from build123d import *

# Parameters (mm, degrees)
ESQUISSE2_R             = 35
ESQUISSE2_R_2           = 5
ESQUISSE2_R_3           = 3.16227766
BASE_EXTRUSION_DEPTH    = 8
ESQUISSE3_R             = 17.492855685
ESQUISSE3_R_2           = 15
BOSS_EXTRU_1_DEPTH      = 20
ESQUISSE4_W             = 72
ESQUISSE4_H             = 33
ENL_V_MAT_EXTRU_2_DEPTH = 57.868268832


with BuildPart() as part:
    # Esquisse2 → Base-Extrusion (new body)
    with BuildSketch(Plane(origin=(0, 0, 0), x_dir=(1, 0, 0), z_dir=(0, 1, 0))):
        Circle(ESQUISSE2_R)
        Circle(ESQUISSE2_R_2, mode=Mode.SUBTRACT)
        with Locations((-28, 0)):
            Circle(ESQUISSE2_R_3, mode=Mode.SUBTRACT)
        with Locations(Location((0, 28, 0), (0, 0, 270))):
            Circle(ESQUISSE2_R_3, mode=Mode.SUBTRACT)
        with Locations((0, -28)):
            Circle(ESQUISSE2_R_3, mode=Mode.SUBTRACT)
        with Locations((28, 0)):
            Circle(ESQUISSE2_R_3, mode=Mode.SUBTRACT)
    extrude(amount=BASE_EXTRUSION_DEPTH)

    # Esquisse3 → Boss.-Extru.1 (add)
    with BuildSketch(Plane(origin=(0, 8, 0), x_dir=(-1, 0, 0), z_dir=(0, 1, 0))):
        Circle(ESQUISSE3_R)
        Circle(ESQUISSE3_R_2, mode=Mode.SUBTRACT)
    extrude(amount=BOSS_EXTRU_1_DEPTH)

    # Esquisse4 → Enlèv. mat.-Extru.2 (cut, through all)
    with BuildSketch(Plane(origin=(0, 0, 0), x_dir=(1, 0, 0), z_dir=(0, 1, 0))):
        with Locations((-1, -16.5)):
            Rectangle(ESQUISSE4_W, ESQUISSE4_H)
    extrude(amount=ENL_V_MAT_EXTRU_2_DEPTH, mode=Mode.SUBTRACT)


with BuildPart() as enl_v_mat_extru_2_kept_piece:
    # of the separate pieces the step leaves, the one the design keeps (enl_v_mat_extru_2_pieces_kept)
    add(part.part.solids().sort_by_distance((35, 0, 0))[0])


solid = enl_v_mat_extru_2_kept_piece.part
The listing builds one solid part. Answer for the finished solid, in the listing's coordinates (mm). A direction names the side the tool comes from. Give positions to 0.01 mm unless a question says otherwise; leave off trailing zeros. Write each loop counter-clockwise with the first axis right and the second up, starting at its lowest first coordinate (ties: lowest second). Pieces come first, ordered by that corner, then holes. Notation, with made-up numbers: (7.25, 69) - (28.25, 69) arc R30 cw to (28.25, 98) - close; hole circle Ø8 at (17, 58). An arc over 180 degrees is marked (long way). One line per question, with ' | ' between items. Start each with the question number.
1. Determine the mould class of faces 4 (the face through (0.38, 17.86, -17.49)), 5 (the face through (0.14, 3.94, -31.16)), 6 (the face through (28.07, 3.94, -3.16)) for opening direction Z: +Z half, -Z half, draft (parallel to the pull), parting line (faces both ways), or undercut.
2. Straight lines are drawn through the part: line 1 (X direction, y = 3, z = -2); line 2 (Y direction, x = 2, z = -22.5); line 3 (X direction, y = 8.25, z = -4.5). For each, find the intervals that lie inside material, in ascending order.
3. Section A-A, the plane x = 0 is taken. Determine the outline of the cut face in (y, z).
4. Section D-D, the plane y = 19.75 is taken. Determine the outline of the cut face in (x, z), then the cut area to 3 significant figures.
5. Given P1, Ø4, axis at x = 4, y = 19.5, coming from the +Z side; P2, Ø8, axis at y = 5.5, z = -28, coming from the -X side; P3, Ø4, axis at y = 9, z = -8.5, coming from the -X side; P4, Ø5.5, axis at x = 0, z = -28, coming from the +Y side, each flat-ended and moving along its own axis, determine where each tip first touches the part or whether it passes through.
6. Section B-B, the plane z = -28 is taken. Determine the outline of the cut face in (x, y).
7. Section C-C, the plane z = -8.5 is taken. Determine the outline of the cut face in (x, y), then the cut area to 3 significant figures.
8. For faces 1 (the face through (-27.93, 3.94, -3.16)), 2 (the face through (0, 8, -18)), 3 (the face through (0, 18, -15)), determine the directions among +Z, -Z, +X, -X, +Y, -Y from which every point of the face is accessible in a straight line to the end or side of a thin tool.
Result:
1) face 4: -Z half | face 5: undercut | face 6: +Z half
2) line 1: x = -34.94 to -30.45, -25.55 to -4.58, 4.58 to 25.55, 30.45 to 34.94 | line 2: y = 0 to 8 | line 3: x = -16.9 to -14.31, 14.31 to 16.9
3) outline: (0, -35) - (8, -35) - (8, -31.16) - (0, -31.16) - close; (0, -24.84) - (8, -24.84) - (8, -17.49) - (28, -17.49) - (28, -15) - (8, -15) - (8, -5) - (0, -5) - close
4) outline: (-17.49, 0) arc R17.49 ccw to (17.49, 0) - (15, 0) arc R15 cw to (-15, 0) - close | area: 127 mm2
5) P1: stops at z = -13.75 | P2: stops at x = -25.48 | P3: stops at x = -34.34 | P4: passes through
6) outline: (-21, 0) - (-3.16, 0) - (-3.16, 8) - (-21, 8) - close; (3.16, 0) - (21, 0) - (21, 8) - (3.16, 8) - close
7) outline: (-33.95, 0) - (33.95, 0) - (33.95, 8) - (15.29, 8) - (15.29, 28) - (12.36, 28) - (12.36, 8) - (-12.36, 8) - (-12.36, 28) - (-15.29, 28) - (-15.29, 8) - (-33.95, 8) - close | area: 660 mm2
8) face 1: +Z, +Y, -Y | face 2: -Z, +Y | face 3: +Z, +Y
